```python
from build123d import *

# Parameters (mm, degrees)
SKETCH1_W           = 12
SKETCH1_H           = 12
SKETCH1_R           = 2
BOSS_EXTRUDE2_DEPTH = 1
BOSS_EXTRUDE5_DEPTH = 15
SKETCH4_R           = 1.2
BOSS_EXTRUDE6_DEPTH = 5


with BuildPart() as part:
    # Sketch1 → Boss-Extrude2 (new body)
    with BuildSketch(Plane(origin=(0, 0, 0), x_dir=(1, 0, 0), z_dir=(0, 1, 0))):
        with Locations((-5.898996881, 2.563822752)):
            Rectangle(SKETCH1_W, SKETCH1_H)
        with Locations((-5.898996881, 2.563822752)):
            Circle(SKETCH1_R, mode=Mode.SUBTRACT)
    extrude(amount=BOSS_EXTRUDE2_DEPTH)

    # Sketch3 → Boss-Extrude5 (add)
    with BuildSketch(Plane(origin=(0, 1, 0), x_dir=(1, 0, 0), z_dir=(0, 1, 0))):
        Polygon((-12.898996881, -4.436177248), (-12.898996881, 0.92811169), (-11.898996881, 0.563822752), (-11.898996881, -3.436177248), (0.101003119, -3.436177248), (0.101003119, 8.563822752), (-11.898996881, 8.563822752), (-11.898996881, 4.563822752), (-12.898996881, 4.800920569), (-12.898996881, 9.563822752), (1.101003119, 9.563822752), (1.101003119, -4.436177248), align=None)
    extrude(amount=-BOSS_EXTRUDE5_DEPTH)

    # Sketch4 → Boss-Extrude6 (add)
    with BuildSketch(Plane(origin=(0, 1, 0), x_dir=(1, 0, 0), z_dir=(0, 1, 0))):
        with Locations((-9.128696242, 5.793522112)):
            Circle(SKETCH4_R)
        with Locations((-2.66929752, 5.793522112)):
            Circle(SKETCH4_R)
        with Locations((-2.66929752, -0.665876609)):
            Circle(SKETCH4_R)
        with Locations((-9.128696242, -0.665876609)):
            Circle(SKETCH4_R)
    extrude(amount=BOSS_EXTRUDE6_DEPTH)


solid = part.part
```
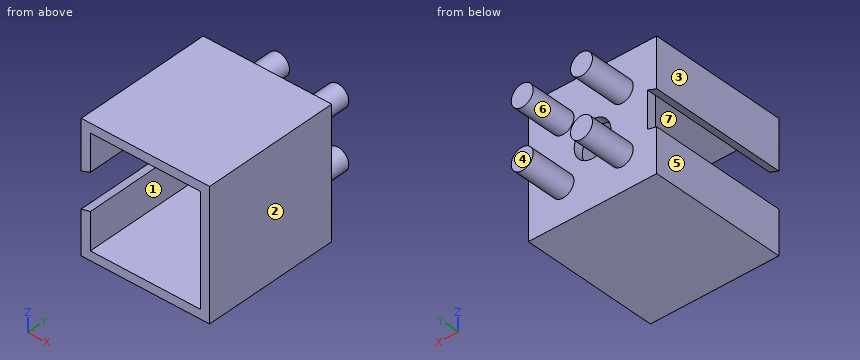
Verification items for the finished model (mm, model axes). Face numbers are marked on the shaded views. A direction names the side the tool comes from. Coordinates: 2 decimals unless noted, no trailing zeros. Loops run counter-clockwise (first coordinate to the right, second up) from the corner with the lowest first, then second, coordinate; pieces in that order, holes last. Notation, with made-up numbers: (-26, 68) -> (2, 68) arc R12 ccw to (2, 76) -> close; hole circle Ø7 at (3.25, 27.5). An arc over 180 degrees is marked (long way). Put each result on its own line as item: value.
1. Section check D-D, the plane x = -11.5. Record the boundary of the cut face in (y, z).
Result set:
outline: (-14, -9.56) -> (1, -9.56) -> (1, 4.44) -> (-14, 4.44) -> (-14, 3.44) -> (0, 3.44) -> (0, -8.56) -> (-14, -8.56) -> close
2. Gauge pin test, flat ends, axial feed: P1, Ø3.5, axis at y = -6, z = -1, coming from the -X side; P2, Ø2, axis at x = -4.5, z = -3, coming from the +Y side; P3, Ø6, axis at x = -3, z = -2, coming from the -Y side. Record the tip position at first contact, or that the pin passes through.
Result set:
P1: stops at x = -12.9
P2: stops at y = 1
P3: stops at y = 0
3. Mould release check, pull along X, two halves, no side actions. Record for the marked faces 1, 2, 3 and 4: pulls with the +X half, pulls with the -X half, needs draft (parallel to the pull), parting line crosses it, or undercut.
Result set:
face 1: undercut
face 2: pulls with the +X half
face 3: pulls with the -X half
face 4: needs draft
4. Tool access check on the marked faces 5, 6 and 7. Record the directions out of +Z, -Z, +X, -X, +Y, -Y that give a thin tool (end or side, any length) a straight path to the whole face; none if there is none.
Result set:
face 5: +Z, -Z, -X, +Y, -Y
face 6: +Y
face 7: -Y
5. Section check A-A, the plane y = -4.25. Record the boundary of the cut face in (x, z), then the cut area to 3 significant figures.
Result set:
outline: (-12.9, -9.56) -> (1.1, -9.56) -> (1.1, 4.44) -> (-12.9, 4.44) -> (-12.9, -0.93) -> (-11.9, -0.56) -> (-11.9, 3.44) -> (0.1, 3.44) -> (0.1, -8.56) -> (-11.9, -8.56) -> (-11.9, -4.56) -> (-12.9, -4.8) -> close
area: 48.1 mm^2
6. Section check B-B, the plane x = -4.25. Record the boundary of the cut face in (y, z), then the cut area to 3 significant figures.
Result set:
outline: (-14, -9.56) -> (1, -9.56) -> (1, -3.7) -> (0, -3.7) -> (0, -8.56) -> (-14, -8.56) -> close; (-14, 3.44) -> (0, 3.44) -> (0, -1.43) -> (1, -1.43) -> (1, 4.44) -> (-14, 4.44) -> close
area: 39.7 mm^2
7. Section check C-C, the plane z = 2.25. Record the boundary of the cut face in (x, y).
Result set:
outline: (-12.9, -14) -> (-11.9, -14) -> (-11.9, 0) -> (0.1, 0) -> (0.1, -14) -> (1.1, -14) -> (1.1, 1) -> (-12.9, 1) -> close
8. Thickness scan on line 1 (X direction, y = -0.5, z = -0.5); line 2 (Z direction, x = -2.25, y = -6); line 3 (Z direction, x = -2.75, y = 2.5). Record the ranges inside material, lowest first.
Result set:
line 1: x = -12.9 to -11.9, 0.1 to 1.1
line 2: z = -9.56 to -8.56, 3.44 to 4.44
line 3: z = -6.99 to -4.6, -0.53 to 1.86
